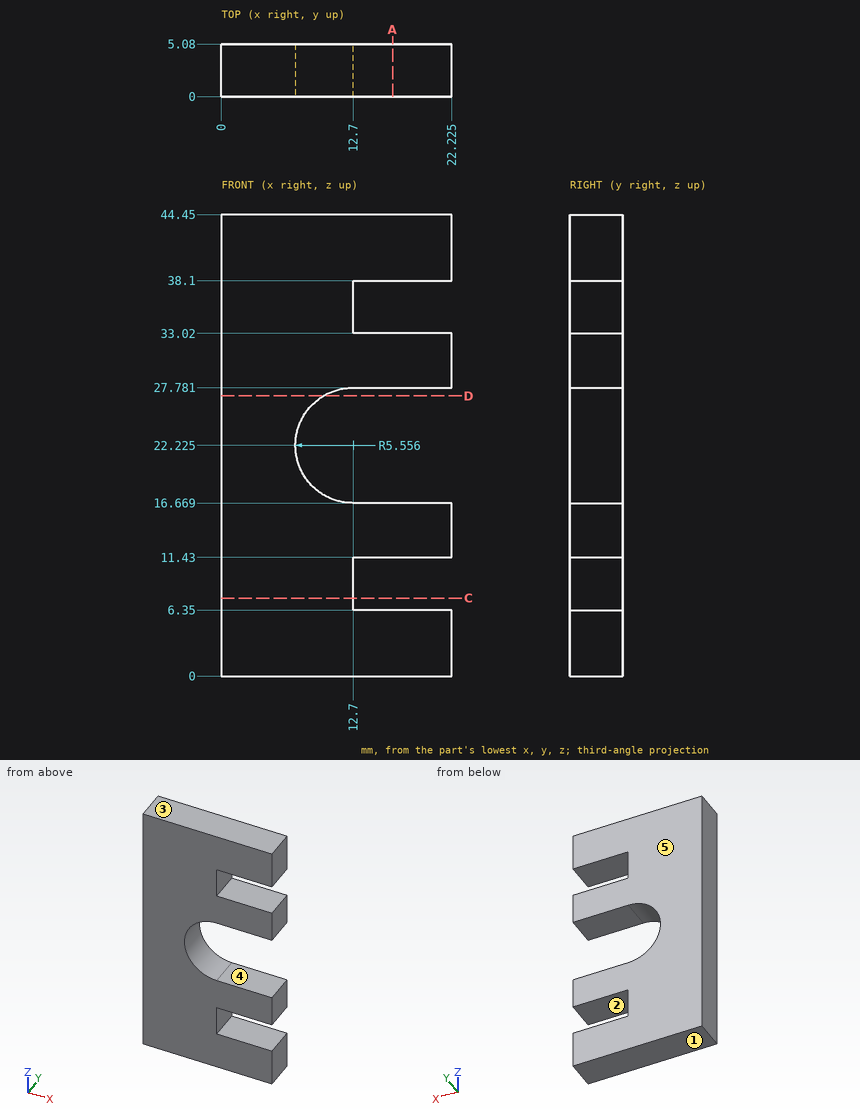
Verification items for this drawing (mm, ordinates from the low corner). A direction names the side the tool comes from. Coordinates: 2 decimals unless noted, no trailing zeros. Loops run counter-clockwise (first coordinate to the right, second up) from the corner with the lowest first, then second, coordinate; pieces in that order, holes last. Notation, with made-up numbers: (50, 6) - (61, 6) arc R28 cw to (61, 45) - close; hole circle Ø3 at (58.25, 21.5). An arc over 180 degrees is marked (long way). Answer as a JSON object with one key per item and string values.
(1) Cross-section at D-D, the plane z = 27. Record the boundary of the cut face in (x, y).
Response:
{"outline": "(0, 0) - (9.86, 0) - (9.86, 5.08) - (0, 5.08) - close"}
(2) Scan lines: line 1 along Z through (x, y) = (13.5, 0.45); line 2 along X through (y, z) = (3.6, 34); line 3 along Z through (x, y) = (8.75, 3.5). Record each from-to range of solid material in increasing order.
Response:
{"line 1": "z = 0 to 6.35, 11.43 to 16.67, 27.78 to 33.02, 38.1 to 44.45", "line 2": "x = 0 to 12.7", "line 3": "z = 0 to 18.32, 26.13 to 44.45"}
(3) Cross-section at A-A, the plane x = 16.5. Record the boundary of the cut face in (y, z), then the cut area to 3 significant figures.
Response:
{"outline": "(0, 0) - (5.08, 0) - (5.08, 6.35) - (0, 6.35) - close; (0, 11.43) - (5.08, 11.43) - (5.08, 16.67) - (0, 16.67) - close; (0, 27.78) - (5.08, 27.78) - (5.08, 33.02) - (0, 33.02) - close; (0, 38.1) - (5.08, 38.1) - (5.08, 44.45) - (0, 44.45) - close", "area": "118 mm²"}
(4) Mould release check, pull along Z, two halves, no side actions. Record for the marked faces 3, 4 and 5: pulls with the +Z half, pulls with the -Z half, needs draft (parallel to the pull), parting line crosses it, or undercut.
Response:
{"face 3": "pulls with the +Z half", "face 4": "undercut", "face 5": "needs draft"}
(5) Cross-section at C-C, the plane z = 7.5. Record the boundary of the cut face in (x, y), then the cut area to 3 significant figures.
Response:
{"outline": "(0, 0) - (12.7, 0) - (12.7, 5.08) - (0, 5.08) - close", "area": "64.5 mm²"}
(6) Access from +Z, -Z, +X, -X, +Y, -Y to the whole of each face (thin tool, end or side, straight path). Record for the marked faces 1 and 2.
Response:
{"face 1": "-Z, +X, -X, +Y, -Y", "face 2": "+X, +Y, -Y"}
